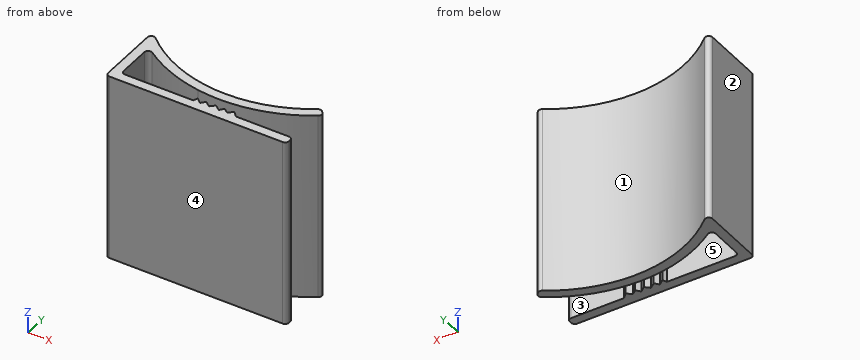
from build123d import *

# Parameters (mm, degrees)
SALIENTE_EXTRUIR1_DEPTH = 25


with BuildPart() as part:
    # Croquis1 → Saliente-Extruir1 (new body)
    with BuildSketch(Plane.XY):
        with BuildLine():
            Line((0.5, 0), (23.5, 0))
            ThreePointArc((23.5, 0), (23.853553391, 0.146446609), (24, 0.5))
            Line((24, 0.5), (24, 0.75))
            ThreePointArc((24, 0.75), (23.853553391, 1.103553391), (23.5, 1.25))
            Line((23.5, 1.25), (16.47782129, 1.25))
            Line((16.47782129, 1.25), (15.856313475, 1.900076822))
            Line((15.856313475, 1.900076822), (15.255148566, 1.325331382))
            Line((15.255148566, 1.325331382), (14.640350544, 1.812303006))
            Line((14.640350544, 1.812303006), (14.194959378, 1.25))
            Line((14.194959378, 1.25), (13.485056051, 1.812303006))
            Line((13.485056051, 1.812303006), (12.896905521, 1.25))
            Line((12.896905521, 1.25), (12.187002195, 1.812303006))
            Line((12.187002195, 1.812303006), (11.72060446, 1.25))
            Line((11.72060446, 1.25), (11.042675201, 1.812303006))
            Line((11.042675201, 1.812303006), (10.797993302, 1.25))
            Line((10.797993302, 1.25), (1.75, 1.25))
            ThreePointArc((1.75, 1.25), (1.396446609, 1.396446609), (1.25, 1.75))
            Line((1.25, 1.75), (1.25, 6.004934433))
            ThreePointArc((1.25, 6.004934433), (1.517138688, 6.44739981), (2.033102437, 6.417066706))
            ThreePointArc((2.033102437, 6.417066706), (5.924204231, 4.346635928), (10.180078199, 3.199947857))
            ThreePointArc((10.180078199, 3.199947857), (17.440764487, 3.465174135), (24.103823344, 6.361992565))
            ThreePointArc((24.103823344, 6.361992565), (24.319661393, 6.719764128), (24.188505071, 7.116481375))
            Line((24.188505071, 7.116481375), (24.015976281, 7.301546958))
            ThreePointArc((24.015976281, 7.301546958), (23.706531625, 7.457420718), (23.370061121, 7.374715069))
            ThreePointArc((23.370061121, 7.374715069), (11.830432965, 4.274140818), (0.835139338, 8.951757379))
            ThreePointArc((0.835139338, 8.951757379), (0.296984814, 9.037632425), (0, 8.580702634))
            Line((0, 8.580702634), (0, 0.5))
            ThreePointArc((0, 0.5), (0.146446609, 0.146446609), (0.5, 0))
        make_face()
    extrude(amount=SALIENTE_EXTRUIR1_DEPTH)


solid = part.part
The model under review builds one solid part; all positions refer to its coordinate system, in mm. Face numbers are marked on the shaded views. A direction names the side the tool comes from. Give positions to 0.01 mm unless a question says otherwise; leave off trailing zeros. Write each loop counter-clockwise with the first axis right and the second up, starting at its lowest first coordinate (ties: lowest second). Pieces come first, ordered by that corner, then holes.
1. Draft analysis for pull direction X (two halves, no side actions). For the marked faces 1, 2 and 3, state which applies: +X half, -X half, draft (parallel to the pull), parting line (faces both ways), or undercut.
2. Add section C-C, the plane x = 18.5. Write out the cut boundary in (y, z).
3. Add section A-A, the plane x = 5. Write out the cut boundary in (y, z).
4. Tool access review of the marked faces 4 and 5: name each direction out of +Z, -Z, +X, -X, +Y, -Y from which nothing blocks a thin tool from reaching the whole face with its end or side.
5. Wall thickness on L1, parallel to Y at x = 7.25, z = 9.5; L2, parallel to Y at x = 8, z = 2.5; L3, parallel to X at y = 2.5, z = 11: over which ranges is each line inside the solid? List them lowest first.
6. Add section D-D, the plane y = 8.25. Write out the cut boundary in (x, z), plus the area to 3 significant figures.
7. For P1, Ø10, axis at x = 6.5, z = 7, coming from the +Y side; P2, Ø7.5, axis at x = 21, z = 18.5, coming from the +Y side; P3, Ø1, axis at x = 4.5, y = 3.5, coming from the -Z side; P4, Ø4.5, axis at y = 4, z = 16, coming from the +X side, all flat-tipped, find the tip position at first contact; note any pin that passes through.
8. Add section B-B, the plane z = 18.5. Write out the cut boundary in (x, y).
Worked answers:
1. face 1: undercut
1. face 2: -X half
1. face 3: draft
2. outline: (0, 0) - (1.25, 0) - (1.25, 25) - (0, 25) - close; (3.74, 0) - (5.04, 0) - (5.04, 25) - (3.74, 25) - close
3. outline: (0, 0) - (1.25, 0) - (1.25, 25) - (0, 25) - close; (4.74, 0) - (6.12, 0) - (6.12, 25) - (4.74, 25) - close
4. face 4: +Z, -Z, +X, -X, -Y
4. face 5: +Z, -Z
5. L1: y = 0 to 1.25, 3.88 to 5.19
5. L2: y = 0 to 1.25, 3.66 to 4.96
5. L3: x = 0 to 1.25
6. outline: (0, 0) - (1.66, 0) - (1.66, 25) - (0, 25) - close
6. area: 41.5 mm2
7. P1: stops at y = 8.38
7. P2: stops at y = 7.46
7. P3: passes through
7. P4: stops at x = 23.94
8. outline: (0, 0.5) arc R0.5 ccw to (0.5, 0) - (23.5, 0) arc R0.5 ccw to (24, 0.5) - (24, 0.75) arc R0.5 ccw to (23.5, 1.25) - (16.48, 1.25) - (15.86, 1.9) - (15.26, 1.33) - (14.64, 1.81) - (14.19, 1.25) - (13.49, 1.81) - (12.9, 1.25) - (12.19, 1.81) - (11.72, 1.25) - (11.04, 1.81) - (10.8, 1.25) - (1.75, 1.25) arc R0.5 cw to (1.25, 1.75) - (1.25, 6) arc R0.5 cw to (2.03, 6.42) arc R19.56 ccw to (24.1, 6.36) arc R0.5 ccw to (24.19, 7.12) - (24.02, 7.3) arc R0.5 ccw to (23.37, 7.37) arc R18.31 cw to (0.84, 8.95) arc R0.5 ccw to (0, 8.58) - close
